```python
from build123d import *

# Parameters (mm, degrees)
PAD_DEPTH       = 20
CHAMFER_SIZE    = 1
CHAMFER001_SIZE = 2
POCKET_DEPTH    = 15.001


with BuildPart() as part:
    # Sketch → Pad (new body)
    with BuildSketch(Plane.XY):
        Polygon((-7.5, 5), (-7.5, -8), (7.5, -8), (7.5, 5), (4.5, 5), (4.5, -5), (-4.5, -5), (-4.5, 5), align=None)
    extrude(amount=PAD_DEPTH)

    # Chamfer
    chamfer_edges = [part.edges().sort_by_distance(p)[0] for p in [
        (-4.5, 5, 10),
        (4.5, 5, 10),
    ]]
    chamfer(chamfer_edges, length=CHAMFER_SIZE)

    # Chamfer001
    chamfer001_edges = [part.edges().sort_by_distance(p)[0] for p in [
        (0, -8, 20),
        (0, -8, 0),
    ]]
    chamfer(chamfer001_edges, length=CHAMFER001_SIZE)

    # Sketch001 (on Face2 of Chamfer001) → Pocket (cut, through all)
    with BuildSketch(Plane.YZ.offset(7.5)):
        Polygon((-2, 20), (5, 20), (5, 13), align=None)
    extrude(amount=-POCKET_DEPTH, mode=Mode.SUBTRACT)


solid = part.part
```
Input: part model. Units: mm. Frame: model coordinates. A direction names the side the tool comes from. Give positions to 0.01 mm unless a question says otherwise; leave off trailing zeros. Order: outer loops, then holes, each group sorted by start corner. A loop starts at its lowest first (then second) coordinate and runs counter-clockwise, first axis right, second up. Notation, with made-up numbers: (24.25, -16) - (59.25, -16) arc R35 ccw to (59.25, 20) - close; hole circle Ø4 at (4, 62.5). An arc over 180 degrees is marked (long way). Put each result on its own line as item: value.
Item 1: Draft query along X for faces 1 (the flat face through (7.5, -2, 10)), 2 (the flat face through (-4.5, -1, 10)), 3 (the flat face through (0, -7, 19)). Return one class per face: +X half, -X half, draft (parallel to the pull), parting line (faces both ways), or undercut.
Found:
face 1: +X half
face 2: undercut
face 3: draft
Item 2: Section query B-B, the plane z = 16. Return loops of the section in (x, y), then the cut area to 3 significant figures.
Found:
outline: (-7.5, -8) - (7.5, -8) - (7.5, 2) - (4.5, 2) - (4.5, -5) - (-4.5, -5) - (-4.5, 2) - (-7.5, 2) - close
area: 87.0 mm^2
Item 3: Contact query for flat-ended pins moving along their axis: pin 1 (3 mm diameter, centred on x = -2.5, y = 0, fed in from -Z); pin 2 (4.5 mm diameter, centred on x = 2, z = 8.5, fed in from +Y). Output: stop coordinate, or through.
Found:
pin 1: passes through
pin 2: stops at y = -5
Item 4: Access query for faces 4 (the flat face through (0, -5, 10)), 5 (the flat face through (-0.1, -5.3, 20)). Directions: +Z, -Z, +X, -X, +Y, -Y. A direction counts if a zero-diameter tool reaches every point of the face in a straight line with its end or side. Return the directions, or none.
Found:
face 4: +Z, -Z, +Y
face 5: +Z, +X, -X, +Y, -Y
Item 5: Ray query, L1, parallel to X at y = -4.5, z = 3; L2, parallel to Y at x = -2, z = 1.5; L3, parallel to Y at x = 0.75, z = 13.5. Return the intervals inside material, ascending. Write a range as from..to.
Found:
L1: x = -7.5..-4.5, 4.5..7.5
L2: y = -7.5..-5
L3: y = -8..-5
Item 6: Section query A-A, the plane y = 3.75. Return loops of the section in (x, z), then the cut area to 3 significant figures.
Found:
outline: (-7.5, 0) - (-4.5, 0) - (-4.5, 14.25) - (-7.5, 14.25) - close; (4.5, 0) - (7.5, 0) - (7.5, 14.25) - (4.5, 14.25) - close
area: 85.5 mm^2
Item 7: Section query D-D, the plane y = -0.75. Return loops of the section in (x, z), then the cut area to 4 significant figures.
Found:
outline: (-7.5, 0) - (-4.5, 0) - (-4.5, 18.75) - (-7.5, 18.75) - close; (4.5, 0) - (7.5, 0) - (7.5, 18.75) - (4.5, 18.75) - close
area: 112.5 mm^2
Item 8: Section query C-C, the plane x = -5.75. Return loops of the section in (y, z), then the cut area to 4 significant figures.
Found:
outline: (-8, 2) - (-6, 0) - (5, 0) - (5, 13) - (-2, 20) - (-6, 20) - (-8, 18) - close
area: 231.5 mm^2
